```python
from build123d import *

# Parameters (mm, degrees)
SZKIC2_R                    = 29
DODANIE_WYCI_GNI_CIE2_DEPTH = 23.5
SZKIC3_R                    = 3
WYTNIJ_WYCI_GNI_CIE1_DEPTH  = 23.5
ZAOKR_GLENIE1_R             = 4
DODANIE_WYCI_GNI_CIE3_REACH = 82
WYTNIJ_WYCI_GNI_CIE2_DEPTH  = 23.5


with BuildPart() as part:
    # Szkic2 → Dodanie-wyciągnięcie2 (new body)
    with BuildSketch(Plane(origin=(0, 0, 0), x_dir=(0, 0, -1), z_dir=(1, 0, 0))):
        with BuildLine():
            Line((-60, -6.5), (60, -6.5))
            Line((60, -6.5), (60, 6.5))
            Line((60, 6.5), (36, 6.5))
            Line((36, 6.5), (31, 35.5))
            ThreePointArc((31, 35.5), (0, 66.5), (-31, 35.5))
            Line((-31, 35.5), (-36, 6.5))
            Line((-36, 6.5), (-60, 6.5))
            Line((-60, 6.5), (-60, -6.5))
        make_face()
        with Locations((0, 33.5)):
            Circle(SZKIC2_R, mode=Mode.SUBTRACT)
    extrude(amount=DODANIE_WYCI_GNI_CIE2_DEPTH)

    # Szkic3 → Wytnij-wyciągnięcie1 (cut)
    with BuildSketch(Plane(origin=(0, 6.5, 0), x_dir=(1, 0, 0), z_dir=(0, 1, 0))):
        with Locations((11.75, 50)):
            Circle(SZKIC3_R)
        with Locations((11.75, -50)):
            Circle(SZKIC3_R)
    extrude(amount=-WYTNIJ_WYCI_GNI_CIE1_DEPTH, mode=Mode.SUBTRACT)

    # Zaokrąglenie1
    zaokr_glenie1_edges = [part.edges().sort_by_distance(p)[0] for p in [
        (11.75, 6.5, -36),
        (11.75, 6.5, 36),
    ]]
    fillet(zaokr_glenie1_edges, radius=ZAOKR_GLENIE1_R)

    # Szkic4 → Dodanie-wyciągnięcie3 (add, up to next)
    with BuildSketch(Plane(origin=(0, 73.5, 0), x_dir=(-1, 0, 0), z_dir=(0, -1, 0)), mode=Mode.PRIVATE) as dodanie_wyci_gni_cie3_sk1:
        Polygon((0, 60), (0, 39.369362474), (0, 35.427522011), (0, 31), (0, -31), (0, -35.427522011), (0, -39.369362474), (0, -60), (-2, -60), (-2, -58), (-2, 58), (-2, 60), align=None)
    dodanie_wyci_gni_cie3_tool1 = extrude(dodanie_wyci_gni_cie3_sk1.sketch, amount=DODANIE_WYCI_GNI_CIE3_REACH, mode=Mode.PRIVATE) - part.part
    add(dodanie_wyci_gni_cie3_tool1.solids().sort_by_distance((1, 73.5, 0))[0])
    # Szkic4 → Dodanie-wyciągnięcie3 (add, up to next)
    with BuildSketch(Plane(origin=(0, 73.5, 0), x_dir=(-1, 0, 0), z_dir=(0, -1, 0)), mode=Mode.PRIVATE) as dodanie_wyci_gni_cie3_sk2:
        Polygon((-23.5, 39.369362474), (-23.5, 60), (-21.5, 60), (-21.5, 58), (-21.5, -58), (-21.5, -60), (-23.5, -60), (-23.5, -39.369362474), (-23.5, -35.427522011), (-23.5, -31), (-23.5, 31), (-23.5, 35.427522011), align=None)
    dodanie_wyci_gni_cie3_tool2 = extrude(dodanie_wyci_gni_cie3_sk2.sketch, amount=DODANIE_WYCI_GNI_CIE3_REACH, mode=Mode.PRIVATE) - part.part
    add(dodanie_wyci_gni_cie3_tool2.solids().sort_by_distance((22.5, 73.5, 0))[0])

    # Szkic5 → Wytnij-wyciągnięcie2 (cut)
    with BuildSketch(Plane(origin=(23.5, 0, 0), x_dir=(0, 0, -1), z_dir=(1, 0, 0))):
        Polygon((-60, 73.5), (-60, 9.5), (-58, 9.5), (-39.369362474, 9.5), (-39.369362474, 73.5), align=None)
        with BuildLine():
            Line((-39.369362474, 73.5), (-39.369362474, 9.5))
            ThreePointArc((-39.369362474, 9.5), (-38.725121416, 9.735177499), (-38.383902359, 10.330093083))
            Line((-38.383902359, 10.330093083), (-35.427522011, 27.477099097))
            Line((-35.427522011, 27.477099097), (-35.427522011, 73.5))
            Line((-35.427522011, 73.5), (-39.369362474, 73.5))
        make_face()
        with BuildLine():
            Line((-31, 73.5), (-31, 49.464240044))
            ThreePointArc((-31, 49.464240044), (0, 69.5), (31, 49.464240044))
            Line((31, 49.464240044), (31, 73.5))
            Line((31, 73.5), (-31, 73.5))
        make_face()
        with BuildLine():
            Line((-35.427522011, 73.5), (-35.427522011, 27.477099097))
            Line((-35.427522011, 27.477099097), (-33.998985816, 35.762609032))
            ThreePointArc((-33.998985816, 35.762609032), (-33.213712716, 42.769751553), (-31, 49.464240044))
            Line((-31, 49.464240044), (-31, 73.5))
            Line((-31, 73.5), (-35.427522011, 73.5))
        make_face()
        with BuildLine():
            Line((35.427522011, 73.5), (35.427522011, 27.477099097))
            Line((35.427522011, 27.477099097), (38.383902359, 10.330093083))
            ThreePointArc((38.383902359, 10.330093083), (38.725121416, 9.735177499), (39.369362474, 9.5))
            Line((39.369362474, 9.5), (39.369362474, 73.5))
            Line((39.369362474, 73.5), (35.427522011, 73.5))
        make_face()
        with BuildLine():
            Line((31, 73.5), (31, 49.464240044))
            ThreePointArc((31, 49.464240044), (33.213712716, 42.769751553), (33.998985816, 35.762609032))
            Line((33.998985816, 35.762609032), (35.427522011, 27.477099097))
            Line((35.427522011, 27.477099097), (35.427522011, 73.5))
            Line((35.427522011, 73.5), (31, 73.5))
        make_face()
        Polygon((39.369362474, 73.5), (39.369362474, 9.5), (58, 9.5), (60, 9.5), (60, 73.5), align=None)
    extrude(amount=-WYTNIJ_WYCI_GNI_CIE2_DEPTH, mode=Mode.SUBTRACT)


solid = part.part
```
The listing builds one solid part. Answer for the finished solid, in the listing's coordinates (mm). A direction names the side the tool comes from. Round coordinates to 2 decimals unless told otherwise and drop trailing zeros. Loops run counter-clockwise (first coordinate to the right, second up) from the corner with the lowest first, then second, coordinate; pieces in that order, holes last. Notation, with made-up numbers: (0.25, 27.25) -> (29.25, 27.25) arc R26 ccw to (29.25, 60.25) -> close; hole circle Ø6 at (27.5, 72.25). An arc over 180 degrees is marked (long way). Use one line per item in the form item = value.
1. The part is cut by section D-D on y = 40. Determine the outline of the cut face in (x, z), and give its area (3 significant figures).
Answer key:
outline = (0, -33.7) -> (2, -33.7) -> (2, -30.67) -> (21.5, -30.67) -> (21.5, -33.7) -> (23.5, -33.7) -> (23.5, -28.26) -> (0, -28.26) -> close; (0, 28.26) -> (23.5, 28.26) -> (23.5, 33.7) -> (21.5, 33.7) -> (21.5, 30.67) -> (2, 30.67) -> (2, 33.7) -> (0, 33.7) -> close
area = 137 mm²
2. Flat-ended cylindrical pins translate along their axes: pin 1 Ø2 at (x, z) = (9, -28) entering from +Y; pin 2 Ø0.6 at (x, z) = (1, 49.5) entering from +Y; pin 3 Ø6 at (x, y) = (15.5, 40) entering from +Z; pin 4 Ø8 at (y, z) = (56, -10) entering from +X. Find the tip coordinate at first contact, or state that the pin passes through.
Answer key:
pin_1 = 50.73
pin_2 = 9.5
pin_3 = 30.96
pin_4 = through
3. The part is cut by section A-A on x = 11.75. Determine the outline of the cut face in (y, z).
Answer key:
outline = (-6.5, -60) -> (6.5, -60) -> (6.5, -53) -> (-6.5, -53) -> close; (-6.5, -47) -> (6.5, -47) -> (6.5, -39.37) arc R4 cw to (9.82, -35.43) -> (35.5, -31) arc R31 ccw to (35.5, 31) -> (9.82, 35.43) arc R4 cw to (6.5, 39.37) -> (6.5, 47) -> (-6.5, 47) -> close; (-6.5, 53) -> (6.5, 53) -> (6.5, 60) -> (-6.5, 60) -> close; hole circle Ø58 at (33.5, 0)
4. For a pull along Z with two mould halves and no side action, classify faces 1 (the cylindrical face through (11.586, 57.953, -15.59)), 2 (the flat face through (12, 0, -60)), 3 (the flat face through (9, 6.5, -48)) as released by +Z, released by -Z, zero draft, split by the parting line, or undercut.
Answer key:
face_1 = undercut
face_2 = released by -Z
face_3 = zero draft
5. The part is cut by section C-C on x = 20. Determine the outline of the cut face in (y, z), and give its area (3 significant figures).
Answer key:
outline = (-6.5, -60) -> (6.5, -60) -> (6.5, -39.37) arc R4 cw to (9.82, -35.43) -> (35.5, -31) arc R31 ccw to (35.5, 31) -> (9.82, 35.43) arc R4 cw to (6.5, 39.37) -> (6.5, 60) -> (-6.5, 60) -> close; hole circle Ø58 at (33.5, 0)
area = 2,380 mm²
6. The part is cut by section B-B on z = 50. Determine the outline of the cut face in (x, y), and give its area (4 significant figures).
Answer key:
outline = (0, -6.5) -> (8.75, -6.5) -> (8.75, 6.5) -> (2, 6.5) -> (2, 9.5) -> (0, 9.5) -> close; (14.75, -6.5) -> (23.5, -6.5) -> (23.5, 9.5) -> (21.5, 9.5) -> (21.5, 6.5) -> (14.75, 6.5) -> close
area = 239.5 mm²
7. Find the intervals of material crossed by probe 1 along Z at (x, y) = (11.75, -2.25); probe 2 along Y at (x, z) = (14, 0); probe 3 along X at (y, z) = (2, 50), in increasing order. Write a range as [from, to].
Answer key:
probe_1 = [-60, -53], [-47, 47], [53, 60]
probe_2 = [-6.5, 4.5], [62.5, 66.5]
probe_3 = [0, 8.75], [14.75, 23.5]
8. A tool of negligible diameter and unlimited length cuts with its end or side. For faces 4 (the flat face through (21.5, 64, 14)), 5 (the flat face through (11.614, 22.48, -33.245)), 6 (the flat face through (11.614, 22.84, 33.183)), 7 (the flat face through (23.5, 4, 4)), from which of +Z, -Z, +X, -X, +Y, -Y can it reach the whole face along a straight path? Write none if from no direction.
Answer key:
face_4 = +Y
face_5 = -Z, +Y
face_6 = +Z, +Y
face_7 = +Z, -Z, +X, +Y, -Y
